For this review, take the finished solid that the model builds, in its own axes (mm). Round coordinates to 2 decimals unless told otherwise and drop trailing zeros. Loops run counter-clockwise (first coordinate to the right, second up) from the corner with the lowest first, then second, coordinate; pieces in that order, holes last.
1. Consider section B-B on y = 20.5. State the section outline as (x, z) points.
2. Clearance check with flat-ended pins moving along their axes: pin 1 Ø0.8 at (x, y) = (107.5, 17) entering from +Z; pin 2 Ø3 at (x, y) = (96.5, 16.5) entering from -Z. State where each tip first meets the part, or that it passes through.
3. To check wall thickness, follow line 1 along X through (y, z) = (17.5, 4.3); line 2 along X through (y, z) = (17.5, 1.1); line 3 along Y through (x, z) = (28, 1.5). State the ranges of each line that lie inside material, in increasing order.
4. Consider section A-A on x = 29. State the section outline as (y, z) points.
5. Consider section C-C on x = 107.7. State the section outline as (y, z) points, then the cut area to 3 significant figures.
6. Consider section D-D on y = 15. State the section outline as (x, z) points, then the cut area to 3 significant figures.
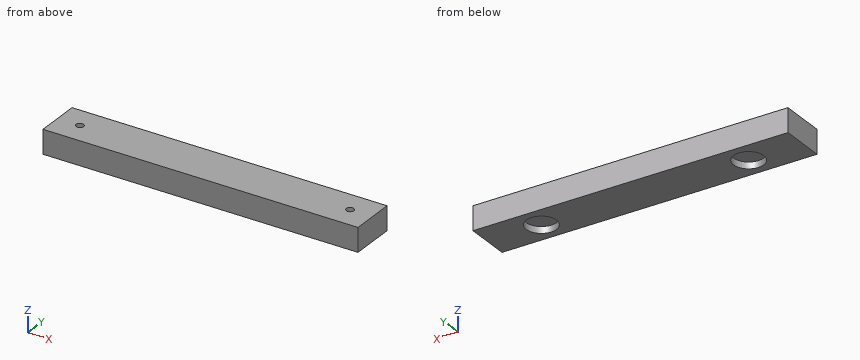
Autodesk Fusion 360 part; units mm, degrees
box "BoitePrimitive1" add length 15 width 105.2 height 8 placed x (0, 1, 0) y (-1, 0, 0) z (0, 0, 1) at (115.2, 10, 0)
hole "Perçage1" at (17.5, 17.5, 8) direction (0, 0, -1) diameter 2.529 depth 6 tip angle 180
hole "Perçage2" at (107.7, 17.5, 8) direction (0, 0, -1) diameter 2.529 depth 6 tip angle 180
hole "Perçage3" at (28, 17.5, 0) direction (0, 0, 1) diameter 10.1 depth 2.2 tip angle 180
hole "Perçage4" at (97.2, 17.5, 0) direction (0, 0, 1) diameter 10.1 depth 2.2 tip angle 180
Resolved:
1. outline: (10, 0) - (23.94, 0) - (23.94, 2.2) - (32.06, 2.2) - (32.06, 0) - (93.14, 0) - (93.14, 2.2) - (101.26, 2.2) - (101.26, 0) - (115.2, 0) - (115.2, 8) - (10, 8) - close
2. pin 1: stops at z = 2
2. pin 2: stops at z = 2.2
3. line 1: x = 10 to 16.24, 18.76 to 106.44, 108.96 to 115.2
3. line 2: x = 10 to 22.95, 33.05 to 92.15, 102.25 to 115.2
3. line 3: y = 10 to 12.45, 22.55 to 25
4. outline: (10, 0) - (12.55, 0) - (12.55, 2.2) - (22.45, 2.2) - (22.45, 0) - (25, 0) - (25, 8) - (10, 8) - close
5. outline: (10, 0) - (25, 0) - (25, 8) - (18.76, 8) - (18.76, 2) - (16.24, 2) - (16.24, 8) - (10, 8) - close
5. area: 105 mm2
6. outline: (10, 0) - (23.61, 0) - (23.61, 2.2) - (32.39, 2.2) - (32.39, 0) - (92.81, 0) - (92.81, 2.2) - (101.59, 2.2) - (101.59, 0) - (115.2, 0) - (115.2, 8) - (10, 8) - close
6. area: 803 mm2
